from build123d import *

# Parameters (mm, degrees)
SKETCH_1_R      = 7.5
EXTRUDE_1_DEPTH = 0.2
SKETCH_2_R      = 4.5
EXTRUDE_2_DEPTH = 0.1
SKETCH_3_R      = 1
EXTRUDE_3_DEPTH = 1
FILLET_1_R      = 0.8
SKETCH_4_R      = 1
EXTRUDE_4_DEPTH = 1
FILLET_2_R      = 0.8
FILLET_3_R      = 0.2


with BuildPart() as part:
    # 草图1 → 凸台-拉伸1 (new body)
    with BuildSketch(Plane(origin=(0, 0, 0), x_dir=(1, 0, 0), z_dir=(0, 1, 0))):
        with Locations(Location((0, 0, 0), (0, 0, 270))):
            Circle(SKETCH_1_R)
    extrude(amount=EXTRUDE_1_DEPTH)

    # 草图2 → 凸台-拉伸2 (add)
    with BuildSketch(Plane(origin=(0, 0.2, 0), x_dir=(1, 0, 0), z_dir=(0, 1, 0))):
        with Locations(Location((0, 0, 0), (0, 0, 270))):
            Circle(SKETCH_2_R)
    extrude(amount=EXTRUDE_2_DEPTH)

    # 草图3 → 凸台-拉伸3 (add)
    with BuildSketch(Plane(origin=(0, 0.2, 0), x_dir=(1, 0, 0), z_dir=(0, 1, 0))):
        with Locations(Location((-5.78398758, -1.72100244, 0), (0, 0, 270))):
            Circle(SKETCH_3_R)
    extrude(amount=EXTRUDE_3_DEPTH)

    # 圆角1
    fillet_1_edges = [part.edges().sort_by_distance(p)[0] for p in [
        (-5.78398758, 1.2, 0.72100244),
    ]]
    fillet(fillet_1_edges, radius=FILLET_1_R)

    # 草图4 → 凸台-拉伸4 (add)
    with BuildSketch(Plane(origin=(0, 0.3, 0), x_dir=(1, 0, 0), z_dir=(0, 1, 0))):
        with Locations(Location((-3.016189843, -0.745176314, 0), (0, 0, 270))):
            Circle(SKETCH_4_R)
    extrude(amount=EXTRUDE_4_DEPTH)

    # 圆角2
    fillet_2_edges = [part.edges().sort_by_distance(p)[0] for p in [
        (-3.016189843, 1.3, -0.254823686),
    ]]
    fillet(fillet_2_edges, radius=FILLET_2_R)

    # 圆角3
    fillet_3_edges = [part.edges().sort_by_distance(p)[0] for p in [
        (-5.78398758, 0.2, 0.72100244),
        (-3.016189843, 0.3, -0.254823686),
    ]]
    fillet(fillet_3_edges, radius=FILLET_3_R - 0.0001)  # a hair under: the kernel refuses the full size


solid = part.part
Can you work these out from the model? Positions are in its coordinate system, mm. A direction names the side the tool comes from. Coordinates: 2 decimals unless noted, no trailing zeros. Order: outer loops, then holes, each group sorted by start corner. A loop starts at its lowest first (then second) coordinate and runs counter-clockwise, first axis right, second up. Notation, with made-up numbers: (84.5, 59.25) - (132.5, 59.25) arc R29 ccw to (132.5, 82.25) - close; hole circle Ø8 at (-11.75, -4.75). An arc over 180 degrees is marked (long way). Answer as a JSON object with one key per item and string values. Group by question number.
Q1. Imagine slicing it at B-B (z = 4.25). Please give me the cut outline in (x, y).
Q2. Will these pins go through, and if not, where does the flat tip stop? P1, Ø5, axis at x = 6, z = -4, coming from the +Y side; P2, Ø7.5, axis at x = 1.5, z = 3, coming from the +Y side.
Q3. I need wall thicknesses on line 1 (Y direction, x = -6.25, z = 0.5); line 2 (X direction, y = 0.4, z = 1.5); line 3 (Y direction, x = -1.25, z = 2.25). Which ranges of each line are inside material? Lowest first, please. Write a range as from..to.
Q4. Imagine slicing it at A-A (x = 0). Please give me the cut outline in (y, z), and give its area (3 significant figures).
Q5. On a 3-axis mill with a long thin cutter (end or side, diameter ignored), from which of +Z, -Z, +X, -X, +Y, -Y can I reach the whole of each face in a straight line? I mean faces 1 (the face through (3.4, 0.2, 3.2)), 2 (the face through (0, 0, 0)). Say none if no direction works.
Determined:
{
 "1": {"outline": "(-6.18, 0) - (6.18, 0) - (6.18, 0.2) - (1.48, 0.2) - (1.48, 0.3) - (-1.48, 0.3) - (-1.48, 0.2) - (-6.18, 0.2) - close"},
 "2": {"P1": "stops at y = 0.2", "P2": "stops at y = 0.3"},
 "3": {"line 1": "y = 0..0.2", "line 2": "x = -6.76..-4.81, -3.71..-2.32", "line 3": "y = 0..0.3"},
 "4": {"outline": "(0, -7.5) - (0.2, -7.5) - (0.2, -4.5) - (0.3, -4.5) - (0.3, 4.5) - (0.2, 4.5) - (0.2, 7.5) - (0, 7.5) - close", "area": "3.90 mm2"},
 "5": {"face 1": "+Y", "face 2": "+Z, -Z, +X, -X, -Y"}
}
